Verification items for the finished model (mm, model axes). Coordinates: 2 decimals unless noted, no trailing zeros. Order: outer loops, then holes, each group sorted by start corner. A loop starts at its lowest first (then second) coordinate and runs counter-clockwise, first axis right, second up. Notation, with made-up numbers: M 4.5,-22.5 L 24.5,-22.5 A22 cw 24.5,-6.5 Z; hole C -32.75,46 d6. An arc over 180 degrees is marked long. Return JSON: item names as keys, results as strings. Group by question number.
1. Section check B-B, the plane x = 13. Record the cut outline in (y, z).
2. Section check A-A, the plane y = 17.5. Record the cut outline in (x, z).
3. Material ranges on line 1 along Z through (x, y) = (0, 28.4); line 2 along X through (y, z) = (0, 164.5); line 3 along Y through (x, z) = (0, 355), recorded low to high.
4. Gauge pin test, flat ends, axial feed: pin 1 (6 mm diameter, centred on x = -5.5, z = 384, fed in from -Y); pin 2 (5 mm diameter, centred on x = 0, z = 372.76, fed in from +Y); pin 3 (4 mm diameter, centred on y = 22.5, z = 70, fed in from +X). Record the tip position at first contact, or that the pin passes through.
Autodesk Inventor part; units mm, degrees
ref_plane "Work Plane9" through (-30.1625, 0, 440) normal (0.2588, 0, 0.9659) x (0, 1, 0)
ref_plane "Work Plane10" through (0, 30.1625, 0) normal (0, 1, 0) x (-1, 0, 0)
ref_plane "Work Plane11" through (0, -30.1625, 0) normal (0, -1, 0) x (1, 0, 0)
sketch "Sketch1" plane through (0, 0, 0) normal (0, 0, 1) x (1, 0, 0)
  circle A0 centre (0, 0) radius 30.1625
  circle A1 centre (0, 0) radius 26.2509
  dimension "d0" = 60.325
  dimension "d2" = 3.9116
extrude "Extrusion1" add sketch "Sketch1" along normal blind 440
sketch "Sketch18" plane through (0, 0, 440) normal (0, 0, 1) x (1, 0, 0)
  circle A0 centre (0, 0) radius 26.2509
  circle A1 centre (0, 0) radius 30.1625
  point P0 (-30.1625, 0)
ref_plane "Work Plane9" through (-30.1625, 0, 440) normal (0.2588, 0, 0.9659) x (0, 1, 0)
sketch "Sketch19" plane through (-30.1625, 0, 440) normal (0.2588, 0, 0.9659) x (0, 1, 0)
  line L0 (-31.6137, -94.9476) -> (64.4261, -94.9476)
  line L1 (64.4261, -94.9476) -> (64.4261, 6.6524)
  line L2 (64.4261, 6.6524) -> (-31.6137, 6.6524)
  line L3 (-31.6137, 6.6524) -> (-31.6137, -94.9476)
  point P0 (0, -143.0151)
  dimension "d61" = 101.6
extrude "Extrusion11" cut sketch "Sketch19" along normal blind 25.4
sketch "Sketch20" plane through (0, 0, 0) normal (0, 0, -1) x (-1, 0, 0)
  circle A0 centre (0, 0) radius 26.2509
  circle A1 centre (0, 0) radius 30.1625
  point P0 (0, 30.1625)
  point P1 (0, -30.1625)
ref_plane "Work Plane10" through (0, 30.1625, 0) normal (0, 1, 0) x (-1, 0, 0)
ref_plane "Work Plane11" through (0, -30.1625, 0) normal (0, -1, 0) x (1, 0, 0)
sketch "Sketch21" plane through (0, 30.1625, 0) normal (0, 1, 0) x (-1, 0, 0)
  line L0 (-3.1444, 432.8221) -> (3.2056, 432.8221)
  line L1 (3.2056, 432.8221) -> (3.2056, 331.2221)
  line L2 (3.2056, 331.2221) -> (-3.1444, 331.2221)
  line L3 (-3.1444, 331.2221) -> (-3.1444, 432.8221)
  line L4 (0.0306, 432.8221) -> (0.0306, 331.2221) construction
  point P0 (0, 0)
  dimension "d64" = 6.35
  dimension "d65" = 101.6
extrude "flat1" cut sketch "Sketch21" against normal blind 0.254
sketch "Sketch22" plane through (0, -30.1625, 0) normal (0, -1, 0) x (1, 0, 0)
  line L0 (-3.1568, 331.2379) -> (3.1932, 331.2379)
  line L1 (3.1932, 331.2379) -> (3.1932, 432.8379)
  line L2 (3.1932, 432.8379) -> (-3.1568, 432.8379)
  line L3 (-3.1568, 432.8379) -> (-3.1568, 331.2379)
  line L4 (0.0182, 432.8379) -> (0.0182, 331.2379) construction
  point P0 (0, 0)
  dimension "d68" = 6.35
  dimension "d69" = 101.6
extrude "flat2" cut sketch "Sketch22" against normal blind 0.254
sketch "Sketch23" plane through (0, -29.9085, 0) normal (0, -1, 0) x (1, 0, 0)
  circle A0 centre (0, 412.7638) radius 1.4603
  circle A1 centre (0, 372.7638) radius 1.4603
  point P0 (-3.1568, 432.7638)
  point P1 (0, 0)
  dimension "d73" = 40
  dimension "d74" = 20
hole "Hole1" at (0, -29.9085, 412.7638) at (0, -29.9085, 372.7638) direction (0, 1, 0) diameter 3.175 end through all
properties part number "2r2scs" material "PVC-Piping"
Answers follow:
{
 "1": {"outline": "M -27.22,0 L -22.81,0 L -22.81,428.43 L -27.22,428.43 Z; M 22.81,0 L 27.22,0 L 27.22,428.43 L 22.81,428.43 Z"},
 "2": {"outline": "M -24.57,0 L -19.57,0 L -19.57,437.16 L -24.57,438.5 Z; M 19.57,0 L 24.57,0 L 24.57,425.33 L 19.57,426.67 Z"},
 "3": {"line 1": "0 to 371.18, 374.35 to 411.18, 414.35 to 431.92", "line 2": "-30.16 to -26.25, 26.25 to 30.16", "line 3": "-29.91 to -26.25, 26.25 to 29.91"},
 "4": {"pin 1": "y = -30", "pin 2": "y = 29.91", "pin 3": "x = 22.13"}
}
